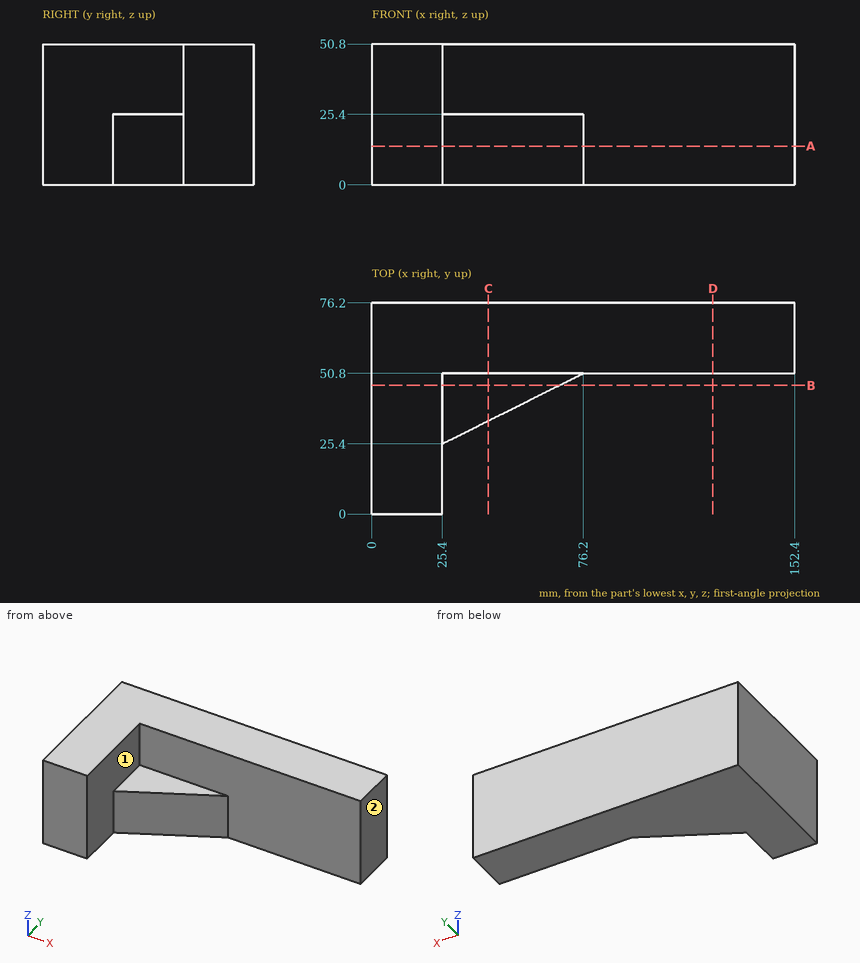
Answer from the drawing. Dimensions are ordinates in mm from the lowest x, y and z of the part. A direction names the side the tool comes from. Round coordinates to 2 decimals unless told otherwise and drop trailing zeros. Write each loop counter-clockwise with the first axis right and the second up, starting at its lowest first coordinate (ties: lowest second). Pieces come first, ordered by that corner, then holes. Notation, with made-up numbers: (64.5, -35.75) -> (105.5, -35.75) arc R14 cw to (105.5, -27.75) -> close; hole circle Ø4 at (-15, 39). An arc over 180 degrees is marked (long way). Write each question's results on one line, items separated by ' | '.
1) The part is cut by section C-C (x = 42). Write down the section's boundary in (y, z), and give its area (3 significant figures).
Findings:
outline: (33.7, 0) -> (76.2, 0) -> (76.2, 50.8) -> (50.8, 50.8) -> (50.8, 25.4) -> (33.7, 25.4) -> close | area: 1,720 mm²
2) Flat-ended cylindrical pins translate along their axes: pin 1 (10 mm diameter, centred on x = 34.5, y = 9, fed in from +Z); pin 2 (20.5 mm diameter, centred on x = 43.5, y = 33.5, fed in from +Z); pin 3 (1 mm diameter, centred on x = 74.5, z = 37, fed in from -Y). Find the tip coordinate at first contact, or state that the pin passes through.
Findings:
pin 1: passes through | pin 2: stops at z = 25.4 | pin 3: stops at y = 50.8
3) The part is cut by section A-A (z = 14). Write down the section's boundary in (x, y).
Findings:
outline: (0, 0) -> (25.4, 0) -> (25.4, 25.4) -> (76.2, 50.8) -> (152.4, 50.8) -> (152.4, 76.2) -> (0, 76.2) -> close
4) Consider line 1 along Y through (x, z) = (127, 8.5); line 2 along X through (y, z) = (50, 40); line 3 along Y through (x, z) = (42.5, 22.5). Determine where each line is inside the solid, lowest interval first. Write a range as [from, to].
Findings:
line 1: y = [50.8, 76.2] | line 2: x = [0, 25.4] | line 3: y = [33.95, 76.2]
5) The part is cut by section D-D (x = 123). Write down the section's boundary in (y, z), and give its area (3 significant figures).
Findings:
outline: (50.8, 0) -> (76.2, 0) -> (76.2, 50.8) -> (50.8, 50.8) -> close | area: 1,290 mm²
6) Which of the six approach directions +Z, -Z, +X, -X, +Y, -Y give full straight-line access (tool end or side, diameter ignored) to the marked faces 1 and 2?
Findings:
face 1: +Z, +X, -Y | face 2: +Z, -Z, +X, +Y, -Y
7) The part is cut by section B-B (y = 46.5). Write down the section's boundary in (x, z).
Findings:
outline: (0, 0) -> (67.6, 0) -> (67.6, 25.4) -> (25.4, 25.4) -> (25.4, 50.8) -> (0, 50.8) -> close
